from build123d import *
from build123d.topology import SkipClean

# Parameters (mm, degrees)
SKETCH1_R           = 19.3
BOSS_EXTRUDE1_DEPTH = 36.7
SKETCH3_R           = 10
BOSS_EXTRUDE2_DEPTH = 5
SKETCH4_R           = 3
BOSS_EXTRUDE3_DEPTH = 15
BOSS_EXTRUDE4_START = -3
SKETCH8_R           = 2.75
BOSS_EXTRUDE4_DEPTH = 15
SKETCH9_R           = 2.75
BOSS_EXTRUDE5_DEPTH = 5
SKETCH5_R           = 1.5
CUT_EXTRUDE1_DEPTH  = 10
CUT_EXTRUDE2_DEPTH  = 10


with BuildPart() as part:
    # Sketch1 → Boss-Extrude1 (new body)
    with BuildSketch(Plane.XY):
        with Locations((-14.127422454, 5.37928778)):
            Circle(SKETCH1_R)
    extrude(amount=BOSS_EXTRUDE1_DEPTH)

    # Sketch3 → Boss-Extrude2 (add)
    with BuildSketch(Plane.XY.offset(36.7)):
        with Locations((-14.127422454, 5.37928778)):
            Circle(SKETCH3_R)
    extrude(amount=BOSS_EXTRUDE2_DEPTH)

    # Sketch4 → Boss-Extrude3 (add)
    with BuildSketch(Plane.XY.offset(41.7)):
        with Locations((-14.127422454, 5.37928778)):
            Circle(SKETCH4_R)
    extrude(amount=BOSS_EXTRUDE3_DEPTH)



with BuildPart() as body_2:
    # Sketch8 → Boss-Extrude4 (new body)
    with BuildSketch(Plane(origin=(0, 24.67928778, 0), x_dir=(1, 0, 0), z_dir=(0, 1, 0)).offset(BOSS_EXTRUDE4_START)):
        with Locations(Location((-26.832117877, -3.04260895, 0), (0, 0, 270))):
            Circle(SKETCH8_R)
    extrude(amount=-BOSS_EXTRUDE4_DEPTH)


with BuildPart() as part_1:
    with SkipClean():  # the faces are left unmerged after this step: merging them gives an invalid solid
        add(part.part)

        add(body_2.part)  # Boss-Extrude5 merges body 2
        # Sketch9 → Boss-Extrude5 (add)
        with BuildSketch(Plane(origin=(0, 21.67928778, 0), x_dir=(1, 0, 0), z_dir=(0, 1, 0))):
            with Locations(Location((-26.832117877, -3.04260895, 0), (0, 0, 329.533131332))):
                Circle(SKETCH9_R)
        extrude(amount=BOSS_EXTRUDE5_DEPTH)

    # Sketch5 → Cut-Extrude1 (cut)
    with SkipClean():  # the faces are left unmerged after this step: merging them gives an invalid solid
        with BuildSketch(Plane.XY.offset(36.7)):
            with Locations((0.862954929, 5.91648973)):
                Circle(SKETCH5_R)
            with Locations((-21.15738061, -7.87136082)):
                Circle(SKETCH5_R)
            with Locations((-22.08784168, 18.092734431)):
                Circle(SKETCH5_R)
        extrude(amount=-CUT_EXTRUDE1_DEPTH, mode=Mode.SUBTRACT)

    # Sketch10 → Cut-Extrude2 (cut)
    with SkipClean():  # the faces are left unmerged after this step: merging them gives an invalid solid
        with BuildSketch(Plane.XY.offset(56.7)):
            Polygon((-86.266834938, 7.87928778), (-15.785734849, 7.87928778), (-12.469110059, 7.87928778), (58.011990031, 7.87928778), (58.011990031, 148.841487959), (-86.266834938, 148.841487959), align=None)
        extrude(amount=-CUT_EXTRUDE2_DEPTH, mode=Mode.SUBTRACT)


solid = part_1.part
Source: CAD feature listing. Evaluate the final solid. Frame: model axes, mm. A direction names the side the tool comes from. Round coordinates to 2 decimals unless told otherwise and drop trailing zeros. Loops run counter-clockwise (first coordinate to the right, second up) from the corner with the lowest first, then second, coordinate; pieces in that order, holes last. Notation, with made-up numbers: (-22, 11) - (-17, 11) arc R28 ccw to (-17, 47) - close; hole circle Ø8 at (-30, 36.25). An arc over 180 degrees is marked (long way). Write item = value, one per line. Start each with the question number.
(1) Pull-direction query (X, two-part tool) for faces 4 (the face through (-27, 26.679, 3)), 5 (the face through (-4.59, 8.38, 39.17)), 6 (the face through (-20.657, 18.543, 31.77)), 7 (the face through (-22, 18, 26.7)); classes: +X half, -X half, draft (parallel to the pull), parting line (faces both ways), or undercut.
(2) Section query B-B, the plane x = -18.5. Output: boundary loops of the cut face in (y, z), plus the area to 3 significant figures.
(3) Section query A-A, the plane y = 22.5. Output: boundary loops of the cut face in (x, z).
(4) Section query C-C, the plane z = 49. Output: boundary loops of the cut face in (x, y).
(5) Ray query, line 1 along X through (y, z) = (6, 20.5); line 2 along Z through (x, y) = (-20, -1); line 3 along X through (y, z) = (6.5, 27). Return the intervals inside material, ascending. Write a range as from..to.
(6) Pin query (flat end, axial travel): pin 1 (10 mm diameter, centred on x = -11.5, z = 49.5, fed in from -Y); pin 2 (0.9 mm diameter, centred on x = -21, y = -7.5, fed in from +Z); pin 3 (12 mm diameter, centred on x = -25.5, y = 5, fed in from +Z). Return the tip coordinate at first contact, or that it passes through.
(7) Section query D-D, the plane y = 3.5. Output: boundary loops of the cut face in (x, z).
(8) Set-up query: faces 1 (the face through (-14, 5, 56.7)), 2 (the face through (-14, 7.879, 52)), 3 (the face through (-21, -8, 26.7)). Return all of +Z, -Z, +X, -X, +Y, -Y with unobstructed straight access to the full face (end or side cutting, diameter ignored); none if empty.
Conclusion:
q1.face_4 = draft
q1.face_5 = parting line
q1.face_6 = undercut
q1.face_7 = undercut
q2.outline = (-13.42, 0) - (24.18, 0) - (24.18, 36.7) - (14.37, 36.7) - (14.37, 41.7) - (-3.61, 41.7) - (-3.61, 36.7) - (-13.42, 36.7) - close
q2.area = 1,470 mm2
q3.outline = circle Ø5.5 at (-26.83, 3.04); (-23.04, 0) - (-5.22, 0) - (-5.22, 36.7) - (-23.04, 36.7) - close
q4.outline = (-15.79, 7.88) arc R3 ccw (long way) to (-12.47, 7.88) - close
q5.line_1 = -33.42..5.16
q5.line_2 = 0..41.7
q5.line_3 = -33.39..-0.52, 2.24..5.14
q6.pin_1 = 2.38
q6.pin_2 = 26.7
q6.pin_3 = 41.7
q7.outline = (-33.34, 0) - (5.08, 0) - (5.08, 36.7) - (-4.31, 36.7) - (-4.31, 41.7) - (-11.79, 41.7) - (-11.79, 56.7) - (-16.47, 56.7) - (-16.47, 41.7) - (-23.95, 41.7) - (-23.95, 36.7) - (-33.34, 36.7) - close
q8.face_1 = +Z, +X, -X, +Y, -Y
q8.face_2 = +Z, +X, -X, +Y
q8.face_3 = +Z
